from build123d import *

# Parameters (mm, degrees)
ESQUISSE1_W        = 34
ESQUISSE1_H        = 34
BOSS_EXTRU_1_DEPTH = 8
BOSS_EXTRU_2_START = 1
ESQUISSE2_R        = 2
BOSS_EXTRU_2_DEPTH = 32


with BuildPart() as part:
    # Esquisse1 → Boss.-Extru.1 (new body)
    with BuildSketch(Plane.XY):
        with Locations((17, 17)):
            Rectangle(ESQUISSE1_W, ESQUISSE1_H)
    extrude(amount=BOSS_EXTRU_1_DEPTH)

    # Esquisse2 → Boss.-Extru.2 (add)
    with BuildSketch(Plane(origin=(0, 0, 0), x_dir=(0, 0, -1), z_dir=(1, 0, 0)).offset(BOSS_EXTRU_2_START)):
        with BuildLine():
            Line((-8, 5.5), (-14, 5.5))
            ThreePointArc((-14, 5.5), (-16.5, 3), (-14, 0.5))
            Line((-14, 0.5), (-8, 0.5))
            Line((-8, 0.5), (-8, 5.5))
        make_face()
        with Locations((-14, 3)):
            Circle(ESQUISSE2_R, mode=Mode.SUBTRACT)
    extrude(amount=BOSS_EXTRU_2_DEPTH)


solid = part.part
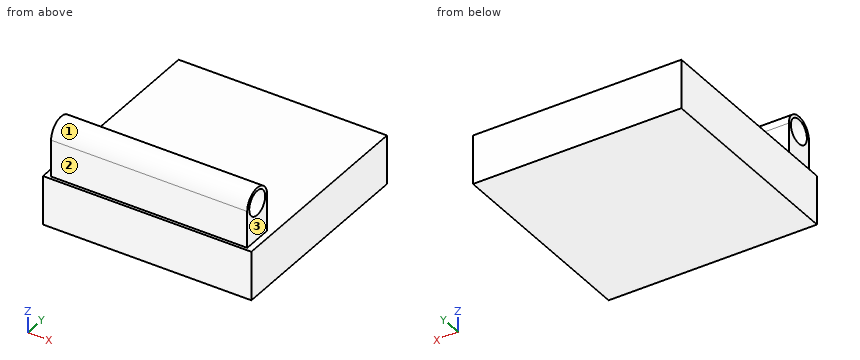
The model under review builds one solid part; all positions refer to its coordinate system, in mm. Face numbers are marked on the shaded views. A direction names the side the tool comes from. Give positions to 0.01 mm unless a question says otherwise; leave off trailing zeros. Write each loop counter-clockwise with the first axis right and the second up, starting at its lowest first coordinate (ties: lowest second). Pieces come first, ordered by that corner, then holes.
1. Add section B-B, the plane x = 4. Write out the cut boundary in (y, z).
2. Wall thickness on L1, parallel to Y at x = 19, z = 14; L2, parallel to Z at x = 9, y = 31; L3, parallel to Y at x = 11, z = 14.75: over which ranges is each line inside the solid? List them lowest first.
3. Add section D-D, the plane y = 28.5. Write out the cut boundary in (x, z).
4. For P1, Ø4, axis at x = 10.5, y = 27.5, coming from the +Z side; P2, Ø4.5, axis at y = 3, z = 14, coming from the +X side; P3, Ø4, axis at x = 10.5, y = 6, coming from the +Z side, all flat-tipped, find the tip position at first contact; note any pin that passes through.
5. Tool access review of the marked faces 1, 2 and 3: name each direction out of +Z, -Z, +X, -X, +Y, -Y from which nothing blocks a thin tool from reaching the whole face with its end or side.
6. Add section C-C, the plane z = 11.5. Write out the cut boundary in (x, y).
7. Add section A-A, the plane y = 3. Write out the cut boundary in (x, z).
Worked answers:
1. outline: (0, 0) - (34, 0) - (34, 8) - (5.5, 8) - (5.5, 14) arc R2.5 ccw to (0.5, 14) - (0.5, 8) - (0, 8) - close; hole circle Ø4 at (3, 14)
2. L1: y = 0.5 to 1, 5 to 5.5
2. L2: z = 0 to 8
2. L3: y = 0.62 to 1.15, 4.85 to 5.38
3. outline: (0, 0) - (34, 0) - (34, 8) - (0, 8) - close
4. P1: stops at z = 8
4. P2: stops at x = 33
4. P3: stops at z = 16.29
5. face 1: +Z, +X, -X
5. face 2: +Z, +X, -X, -Y
5. face 3: +Z, +X, +Y, -Y
6. outline: (1, 0.5) - (33, 0.5) - (33, 5.5) - (1, 5.5) - close
7. outline: (0, 0) - (34, 0) - (34, 8) - (33, 8) - (33, 12) - (1, 12) - (1, 8) - (0, 8) - close; (1, 16) - (33, 16) - (33, 16.5) - (1, 16.5) - close
